from build123d import *

# Parameters (mm, degrees)
BOSS_EXTRU_1_DEPTH      = 10
CONG_1_R                = 0.5
CONG_2_R                = 1
ESQUISSE2_R             = 2.1
ENL_V_MAT_EXTRU_1_DEPTH = 13.661149081102538
ENL_V_MAT_EXTRU_2_DEPTH = 3


with BuildPart() as part:
    # Esquisse1 → Boss.-Extru.1 (new body)
    with BuildSketch(Plane.XY):
        Polygon((-1.176e-14, 10.103135382441117), (-2.578e-14, 4.840000000000001), (3.5, 4.840000000000001), (5.71, 6.983135382441116), (5.71, 8.483135382441116), (2.95, 8.483135382441116), (2.95, 10.103135382441117), align=None)
        Polygon((-3.5, 4.840000000000001), (-2.576e-14, 4.840000000000001), (-1.176e-14, 10.103135382441117), (-2.95, 10.103135382441117), (-2.95, 8.483135382441116), (-5.71, 8.483135382441116), (-5.71, 6.983135382441116), align=None)
    extrude(amount=-BOSS_EXTRU_1_DEPTH)

    # Congé1
    cong_1_edges = [part.edges().sort_by_distance(p)[0] for p in [
        (5.71, 7.733135382441116, 0),
        (4.605, 5.911567691220558, 0),
        (0, 4.840000000000001, 0),
        (-4.605, 5.911567691220558, 0),
        (-5.71, 7.733135382441116, 0),
        (-5.71, 7.733135382441116, -10),
        (-4.605, 5.911567691220558, -10),
        (0, 4.840000000000001, -10),
        (4.605, 5.911567691220558, -10),
        (5.71, 7.733135382441116, -10),
    ]]
    fillet(cong_1_edges, radius=CONG_1_R)

    # Congé2
    # the kernel refuses this fillet: 1 mm, written as the material it takes off along each edge
    with BuildSketch(Plane(origin=(4.71, 7.4063748668930085, -10), x_dir=(1, 0, 0), z_dir=(0, 1, 0))) as cong_2_piece_1:
        with BuildLine():
            CenterArc((0.5, -0.5), 0.5, 0, 90)
            Line((1, -0.5), (1, 0))
            Line((1, 0), (0.5, 0))
        make_face()
    revolve(axis=Axis((4.71, 7.4063748668930085, -10), (0, 0, -1)), revolution_arc=45.87999999999987, mode=Mode.SUBTRACT)
    with BuildSketch(Plane(origin=(-4.710000000000001, 7.40637486689301, -10), x_dir=(-0.6961634275566162, -0.717883334625219, 0), z_dir=(0.717883334625219, -0.6961634275566162, 0))) as cong_2_piece_2:
        with BuildLine():
            CenterArc((0.5, -0.5), 0.5, 0, 90)
            Line((1, -0.5), (1, 0))
            Line((1, 0), (0.5, 0))
        make_face()
    revolve(axis=Axis((-4.710000000000001, 7.40637486689301, -10), (0, 0, -1)), revolution_arc=45.87999999999987, mode=Mode.SUBTRACT)
    with BuildSketch(Plane(origin=(4.71, 7.4063748668930085, 0), x_dir=(0.6961634275566162, -0.717883334625219, 0), z_dir=(-0.717883334625219, -0.6961634275566162, 0))) as cong_2_piece_3:
        with BuildLine():
            CenterArc((0.5, -0.5), 0.5, 0, 90)
            Line((1, -0.5), (1, 0))
            Line((1, 0), (0.5, 0))
        make_face()
    revolve(axis=Axis((4.71, 7.4063748668930085, 0), (0, 0, 1)), revolution_arc=45.87999999999987, mode=Mode.SUBTRACT)
    with BuildSketch(Plane(origin=(-4.710000000000001, 7.40637486689301, 0), x_dir=(-1, 0, 0), z_dir=(0, 1, 0))) as cong_2_piece_4:
        with BuildLine():
            CenterArc((0.5, -0.5), 0.5, 0, 90)
            Line((1, -0.5), (1, 0))
            Line((1, 0), (0.5, 0))
        make_face()
    revolve(axis=Axis((-4.710000000000001, 7.40637486689301, 0), (0, 0, 1)), revolution_arc=45.87999999999987, mode=Mode.SUBTRACT)
    with BuildSketch(Plane(origin=(-5.71, 6.983135382441116, 1.1e-16), x_dir=(0.717883334625219, -0.6961634275566161, 0), z_dir=(0, 0, -1))) as cong_2_piece_5:
        with BuildLine():
            CenterArc((CONG_2_R * 0.423239484452, -CONG_2_R), CONG_2_R, 90.00000000000003, 45.879999999999825)
            Line((-CONG_2_R * 0.294643850173, -CONG_2_R * 0.303836572443), (0, 0))
            Line((0, 0), (CONG_2_R * 0.423239484452, 0))
        make_face()
    extrude(amount=10, mode=Mode.SUBTRACT)
    with BuildSketch(Plane(origin=(5.71, 6.983135382441116, 1.1e-16), x_dir=(-0.7178833346252179, -0.6961634275566172, 0), z_dir=(0, 0, -1))) as cong_2_piece_6:
        with BuildLine():
            CenterArc((CONG_2_R * 0.423239484452, CONG_2_R), CONG_2_R, 224.12000000000015, 45.87999999999994)
            Line((-CONG_2_R * 0.294643850173, CONG_2_R * 0.303836572443), (0, 0))
            Line((0, 0), (CONG_2_R * 0.423239484452, 2e-17))
        make_face()
    extrude(amount=10, mode=Mode.SUBTRACT)

    # Esquisse2 → Enlèv. mat.-Extru.1 (cut, through all)
    with BuildSketch(Plane(origin=(0, 10.103135382441117, 0), x_dir=(1, 0, 0), z_dir=(0, 1, 0))):
        with Locations(Location((0, 5, 0), (0, 0, 270))):
            Circle(ESQUISSE2_R)
    extrude(amount=-ENL_V_MAT_EXTRU_1_DEPTH, mode=Mode.SUBTRACT)

    # Esquisse3 → Enlèv. mat.-Extru.2 (cut)
    with BuildSketch(Plane.XZ.offset(-4.840000000000001)):
        Polygon((0, -9.05), (3.5074028853269765, -7.025), (3.5074028853269774, -2.975), (5e-16, -0.9499999999999995), (-3.5074028853269774, -2.975), (-3.5074028853269774, -7.025000000000001), align=None)
    extrude(amount=-ENL_V_MAT_EXTRU_2_DEPTH, mode=Mode.SUBTRACT)


solid = part.part
Geometry check sheet. Reference: the model listing, model coordinates, mm. A direction names the side the tool comes from. Round coordinates to 2 decimals unless told otherwise and drop trailing zeros. Loops run counter-clockwise (first coordinate to the right, second up) from the corner with the lowest first, then second, coordinate; pieces in that order, holes last. Notation, with made-up numbers: (-14, 4) -> (35, 4) arc R23 ccw to (35, 14) -> close; hole circle Ø2 at (28, 43). An arc over 180 degrees is marked (long way). Answer as a JSON object with one key per item and string values. Group by question number.
Item 1: Cross-section at C-C, the plane y = 9.45. Record the cut outline in (x, z), plus the area to 3 significant figures.
Item 2: Thickness scan on line 1 along X through (y, z) = (8.3, -5); line 2 along X through (y, z) = (8.8, -5); line 3 along Z through (x, y) = (-0.75, 6.9). Record the ranges inside material, lowest first.
Item 3: Cross-section at A-A, the plane z = -4.75. Record the cut outline in (x, y), plus the area to 3 significant figures.
Item 4: Cross-section at D-D, the plane z = -8.25. Record the cut outline in (x, y).
Item 5: Release check for a two-part mould opening along X. For faces 4 (the face through (-4.34, 5.85, -9.85)), 5 (the face through (5.71, 8, -5)), 6 (the face through (1.778, 6.319, -1.977)) record: pulls with the +X half, pulls with the -X half, needs draft (parallel to the pull), parting line crosses it, or undercut.
Item 6: Depth check by flat-ended pin: pin 1 Ø1 at (x, z) = (-1, -3) entering from -Y; pin 2 Ø2.5 at (y, z) = (5.5, -4.5) entering from +X; pin 3 Ø3 at (x, y) = (-1, 9) entering from +Z; pin 4 Ø2.5 at (y, z) = (6, -5.5) entering from -X. Enter the tip coordinate at first touch or a pass-through.
Item 7: Set-up check for faces 1 (the face through (4, 8.483, -5)), 2 (the face through (-3.507, 6, -5)), 3 (the face through (-4, 8.483, -5)): record each of +Z, -Z, +X, -X, +Y, -Y from which the full face is reachable in a straight line by a thin tool's end or side.
Item 8: Cross-section at B-B, the plane x = -1. Record the cut outline in (y, z), plus the area to 3 significant figures.
Determined:
{
 "1": {"outline": "(-2.95, -10) -> (2.95, -10) -> (2.95, 0) -> (-2.95, 0) -> close; hole circle Ø4.2 at (0, -5)", "area": "45.1 mm²"},
 "2": {"line 1": "x = -5.71 to -2.1, 2.1 to 5.71", "line 2": "x = -2.95 to -2.1, 2.1 to 2.95", "line 3": "z = -10 to -8.62, -1.38 to 0"},
 "3": {"outline": "(-5.71, 7.41) arc R1 ccw to (-5.41, 6.69) -> (-3.51, 4.85) -> (-3.51, 7.84) -> (-2.09, 7.84) -> (-2.09, 10.1) -> (-2.95, 10.1) -> (-2.95, 8.48) -> (-5.71, 8.48) -> close; (2.09, 7.84) -> (3.51, 7.84) -> (3.51, 4.85) -> (5.41, 6.69) arc R1 ccw to (5.71, 7.41) -> (5.71, 8.48) -> (2.95, 8.48) -> (2.95, 10.1) -> (2.09, 10.1) -> close", "area": "15.9 mm²"},
 "4": {"outline": "(-5.71, 7.41) arc R1 ccw to (-5.41, 6.69) -> (-3.5, 4.84) -> (-1.39, 4.84) -> (-1.39, 7.84) -> (1.39, 7.84) -> (1.39, 4.84) -> (3.5, 4.84) -> (5.41, 6.69) arc R1 ccw to (5.71, 7.41) -> (5.71, 8.48) -> (2.95, 8.48) -> (2.95, 10.1) -> (-2.95, 10.1) -> (-2.95, 8.48) -> (-5.71, 8.48) -> close"},
 "5": {"face 4": "pulls with the -X half", "face 5": "pulls with the +X half", "face 6": "undercut"},
 "6": {"pin 1": "stops at y = 7.84", "pin 2": "stops at x = 5.46", "pin 3": "stops at z = 0", "pin 4": "stops at x = -5.7"},
 "7": {"face 1": "+Z, -Z, +X, +Y", "face 2": "-Y", "face 3": "+Z, -Z, -X, +Y"},
 "8": {"outline": "(4.84, -9.5) arc R0.5 ccw to (5.34, -10) -> (10.1, -10) -> (10.1, -6.85) -> (7.84, -6.85) -> (7.84, -8.47) -> (4.84, -8.47) -> close; (4.84, -1.53) -> (7.84, -1.53) -> (7.84, -3.15) -> (10.1, -3.15) -> (10.1, 0) -> (5.34, 0) arc R0.5 ccw to (4.84, -0.5) -> close", "area": "23.3 mm²"}
}
